Autodesk Fusion 360 part; units mm, degrees
sketch "Sketch1" plane through (0, 0, 0) normal (0, 0, 1) x (1, 0, 0)
  line L0 (0, 0) -> (40, 0)
  line L1 (40, 0) -> (40, 150)
  line L2 (40, 150) -> (0, 150)
  line L3 (0, 150) -> (0, 0)
  line L4 (17.1, 150) -> (23.3, 150)
  line L5 (23.3, 150) -> (23.3, 157)
  line L6 (23.3, 157) -> (17.1, 157)
  line L7 (17.1, 157) -> (17.1, 150)
  circle A0 centre (20.0369, 161.3) radius 5.7
  circle A1 centre (20, 11.85) radius 6.45
  line L8 (16.1, 0) -> (23.9, 0)
  line L9 (23.9, 0) -> (23.9, 7)
  line L10 (23.9, 7) -> (16.1, 7)
  line L11 (16.1, 7) -> (16.1, 0)
  dimension "d1" = 40
  dimension "d2" = 150
  dimension "d3" = 6.2
  dimension "d4" = 7
  dimension "d5" = 23.3
  dimension "d6" = 11.4
  dimension "d8" = 17
  dimension "d9" = 12.9
  dimension "d11" = 18.3
  dimension "d12" = 20
  dimension "d13" = 7.8
  dimension "d14" = 7
  dimension "d15" = 16.1
extrude "Extrude1" add sketch "Sketch1" along normal blind 12 contours L0 L1 L2 L3 L4 A1 L9 L11 | L2 L4 L5 L7 A0 | L5 L6 L7 A0 | L5 L6 L7 A0
sketch "Sketch2" plane through (0, 0, 12) normal (0, 0, 1) x (-1, 0, 0)
  line L0 (-23.9, 0) -> (-40, 0)
  line L1 (-40, 0) -> (-40, -150)
  line L2 (-40, -150) -> (-23.3, -150)
  line L3 (-23.3, -150) -> (-23.3, -156.6265)
  arc A0 (-23.3, -156.6265) -> (-17.1, -156.4148) centre (-20.0369, -161.3) ccw
  line L4 (-17.1, -156.4148) -> (-17.1, -150)
  line L5 (-17.1, -150) -> (0, -150)
  line L6 (0, -150) -> (0, 0)
  line L7 (0, 0) -> (-16.1, 0)
  line L8 (-16.1, 0) -> (-16.1, -6.7126)
  arc A1 (-23.9, -6.7126) -> (-16.1, -6.7126) centre (-20, -11.85) ccw
  line L9 (-23.9, -6.7126) -> (-23.9, 0)
  line L10 (-4.5, 0) -> (-10.5, 0)
  line L11 (-10.5, 0) -> (-10.5, -150)
  line L12 (-10.5, -150) -> (-4.5, -150)
  line L13 (-4.5, -150) -> (-4.5, 0)
  line L14 (-35.5, 0) -> (-29.5, 0)
  line L15 (-29.5, 0) -> (-29.5, -150)
  line L16 (-29.5, -150) -> (-35.5, -150)
  line L17 (-35.5, -150) -> (-35.5, 0)
  dimension "d18" = 6
  dimension "d19" = 150
  dimension "d20" = 4.5
  dimension "d21" = 6
  dimension "d22" = 150
  dimension "d23" = 4.5
extrude "Extrude2" cut sketch "Sketch2" against normal blind 2.9 contours L0 L2 L14 L15 L16 L17 | L5 L7 L10 L11 L12 L13
fillet "Fillet1" radius 1.1 6 edges at (4.5, 75, 12) (0, 75, 12) (10.5, 75, 12) (29.5, 75, 12) (35.5, 75, 12) (40, 75, 12)
Geometry check sheet. Reference: the model listing, model coordinates, mm. A direction names the side the tool comes from. Round coordinates to 2 decimals unless told otherwise and drop trailing zeros. Loops run counter-clockwise (first coordinate to the right, second up) from the corner with the lowest first, then second, coordinate; pieces in that order, holes last. Notation, with made-up numbers: (49.5, 82.5) - (80.5, 82.5) arc R32 ccw to (80.5, 116.5) - close; hole circle Ø1 at (38.25, 29). An arc over 180 degrees is marked (long way). Write each question's results on one line, items separated by ' | '. Start each with the question number.
Q1. Cross-section at C-C on x = 33.5. Enter the section's corners in (y, z), and give its area (4 significant figures).
Q2. Cross-section at A-A on y = 11.85. Enter the section's corners in (x, z), and give its area (3 significant figures).
Q3. Thickness scan on line 1 (X direction, y = 78.5, z = 11.25); line 2 (X direction, y = 11.85, z = 9.5); line 3 (X direction, y = 61.5, z = 10.5). Record the ranges inside material, lowest first. Write a range as [from, to].
Q4. Release check for a two-part mould opening along Y. For faces 4 (the flat face through (8, 0, 6)), 5 (the flat face through (23.3, 153, 6)), 6 (the flat face through (23.9, 3, 6)), 7 (the flat face through (32, 150, 6)) record: +Y half, -Y half, draft (parallel to the pull), parting line (faces both ways), or undercut.
Q5. Cross-section at B-B on z = 3.75. Enter the section's corners in (x, y).
Q6. Cross-section at D-D on y = 130. Enter the section's corners in (x, z).
Q7. Gauge pin test, flat end, axial feed: P1, Ø1.8, axis at x = 34, y = 88.5, coming from the +Z side. Record the tip position at first contact, or that the pin passes through.
Q8. Access from +Z, -Z, +X, -X, +Y, -Y to the whole of each face (thin tool, end or side, straight path). Record for faces 1 (the flat face through (9, 150, 6)), 2 (the flat face through (16.1, 3, 6)), 3 (the flat face through (8, 74, 9.1)).
Answers below:
1) outline: (0, 0) - (150, 0) - (150, 9.1) - (0, 9.1) - close | area: 1,365 mm²
2) outline: (0, 0) - (13.55, 0) - (13.55, 12) - (11.6, 12) arc R1.1 ccw to (10.5, 10.9) - (10.5, 9.1) - (4.5, 9.1) - (4.5, 10.9) arc R1.1 ccw to (3.4, 12) - (1.1, 12) arc R1.1 ccw to (0, 10.9) - close; (26.45, 0) - (40, 0) - (40, 10.9) arc R1.1 ccw to (38.9, 12) - (36.6, 12) arc R1.1 ccw to (35.5, 10.9) - (35.5, 9.1) - (29.5, 9.1) - (29.5, 10.9) arc R1.1 ccw to (28.4, 12) - (26.45, 12) - close | area: 289 mm²
3) line 1: x = [0.06, 4.44], [10.56, 29.44], [35.56, 39.94] | line 2: x = [0, 4.5], [10.5, 13.55], [26.45, 29.5], [35.5, 40] | line 3: x = [0, 4.5], [10.5, 29.5], [35.5, 40]
4) face 4: -Y half | face 5: undercut | face 6: draft | face 7: undercut
5) outline: (0, 0) - (16.1, 0) - (16.1, 6.71) arc R6.45 cw (long way) to (23.9, 6.71) - (23.9, 0) - (40, 0) - (40, 150) - (23.3, 150) - (23.3, 156.63) arc R5.7 ccw (long way) to (17.1, 156.41) - (17.1, 150) - (0, 150) - close
6) outline: (0, 0) - (40, 0) - (40, 10.9) arc R1.1 ccw to (38.9, 12) - (36.6, 12) arc R1.1 ccw to (35.5, 10.9) - (35.5, 9.1) - (29.5, 9.1) - (29.5, 10.9) arc R1.1 ccw to (28.4, 12) - (11.6, 12) arc R1.1 ccw to (10.5, 10.9) - (10.5, 9.1) - (4.5, 9.1) - (4.5, 10.9) arc R1.1 ccw to (3.4, 12) - (1.1, 12) arc R1.1 ccw to (0, 10.9) - close
7) P1: stops at z = 9.1
8) face 1: +Z, -Z, -X | face 2: +Z, -Z, -Y | face 3: +Z, +Y, -Y
